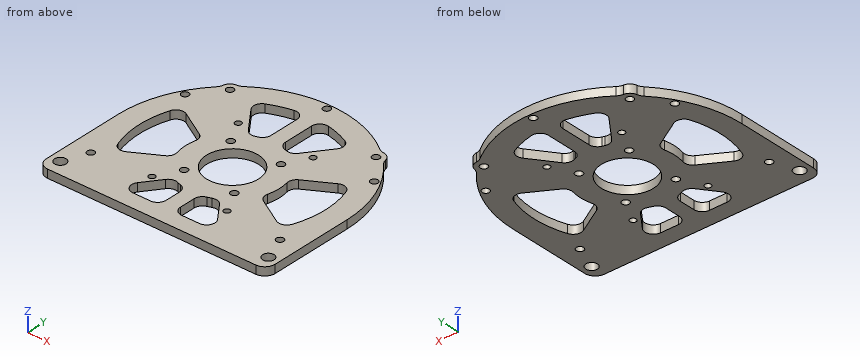
```python
from build123d import *

# Parameters (mm, degrees)
SKETCH_2_R          = 1.25
SKETCH_2_R_2        = 1.75
SKETCH_2_R_3        = 12.5
SKETCH_2_R_4        = 2.55
SKETCH_2_R_5        = 1.5
SKETCH_2_R_6        = 1.55
EXTRUDE_1_DEPTH     = 4
CUT_EXTRUDE_1_DEPTH = 4
FILLET_2_R          = 4
FILLET_3_R          = 4
FILLET_4_R          = 5
SKETCH_4_R          = 1.75
SKETCH_4_R_2        = 1.5
SKETCH_4_R_3        = 2.75
CUT_EXTRUDE_2_DEPTH = 10


with BuildPart() as part:
    # 草图2 → 凸台-拉伸1 (new body)
    with BuildSketch(Plane.XY):
        with BuildLine():
            Line((55, 3), (55, 47.999999928))
            ThreePointArc((55, 47.999999928), (50.85407892, 68.949049075), (39.041357871, 86.739803505))
            ThreePointArc((39.041357871, 86.739803505), (37.739334229, 90.232640986), (34.122629592, 91.135207774))
            ThreePointArc((34.122629592, 91.135207774), (0, 103), (-34.122629592, 91.135207774))
            ThreePointArc((-34.122629592, 91.135207774), (-37.739334229, 90.232640986), (-39.041357871, 86.739803505))
            ThreePointArc((-39.041357871, 86.739803505), (-50.854078907, 68.949049108), (-55, 48))
            Line((-55, 48), (-55, 3))
            Line((-55, 3), (55, 3))
        make_face()
        with Locations((-18, 24)):
            Circle(SKETCH_2_R, mode=Mode.SUBTRACT)
        with Locations((-12.07, 35)):
            Circle(SKETCH_2_R_2, mode=Mode.SUBTRACT)
        with Locations((18, 24)):
            Circle(SKETCH_2_R, mode=Mode.SUBTRACT)
        with Locations((12.07, 35)):
            Circle(SKETCH_2_R_2, mode=Mode.SUBTRACT)
        with Locations((0, 48)):
            Circle(SKETCH_2_R_3, mode=Mode.SUBTRACT)
        with Locations((-12.07, 61)):
            Circle(SKETCH_2_R_2, mode=Mode.SUBTRACT)
        with Locations((-18, 72)):
            Circle(SKETCH_2_R, mode=Mode.SUBTRACT)
        with Locations((12.07, 61)):
            Circle(SKETCH_2_R_2, mode=Mode.SUBTRACT)
        with Locations((18, 72)):
            Circle(SKETCH_2_R, mode=Mode.SUBTRACT)
        with Locations((50, 10)):
            Circle(SKETCH_2_R_4, mode=Mode.SUBTRACT)
        with Locations((45.466333699, 21.75)):
            Circle(SKETCH_2_R_5, mode=Mode.SUBTRACT)
        with Locations((45.466333699, 74.25)):
            Circle(SKETCH_2_R_5, mode=Mode.SUBTRACT)
        with Locations((35.074028853, 87.25)):
            Circle(SKETCH_2_R_6, mode=Mode.SUBTRACT)
        with Locations((-50, 10)):
            Circle(SKETCH_2_R_4, mode=Mode.SUBTRACT)
        with Locations((0, 100.5)):
            Circle(SKETCH_2_R_5, mode=Mode.SUBTRACT)
        with Locations((-45.466333699, 21.75)):
            Circle(SKETCH_2_R_5, mode=Mode.SUBTRACT)
        with Locations((-45.466333699, 74.25)):
            Circle(SKETCH_2_R_5, mode=Mode.SUBTRACT)
        with Locations((-35.074028853, 87.25)):
            Circle(SKETCH_2_R_6, mode=Mode.SUBTRACT)
    extrude(amount=EXTRUDE_1_DEPTH)

    # 草图3 → 切除-拉伸1 (cut)
    with BuildSketch(Plane.XY.offset(4)):
        with BuildLine():
            ThreePointArc((-3.5, 25.773889229), (-7.354360894, 26.735866445), (-10.979461873, 28.360717503))
            Line((-10.979461873, 28.360717503), (-24, 11))
            Line((-24, 11), (-3.5, 11))
            Line((-3.5, 11), (-3.5, 25.773889229))
        make_face()
        with BuildLine():
            Line((-21.175179269, 55.606693298), (-40.502045801, 66.765064893))
            ThreePointArc((-40.502045801, 66.765064893), (-44.635096369, 47.4984557), (-40.070163739, 28.329581794))
            Line((-40.070163739, 28.329581794), (-20.811589784, 39.448524651))
            ThreePointArc((-20.811589784, 39.448524651), (-22.494305888, 47.493835393), (-21.175179269, 55.606693298))
        make_face()
        with BuildLine():
            ThreePointArc((-3.5, 92.500487352), (-13.877512662, 90.425912092), (-23.474999809, 85.966666412))
            Line((-23.474999809, 85.966666412), (-10.084953895, 68.11327186))
            ThreePointArc((-10.084953895, 68.11327186), (-6.874137411, 69.424197414), (-3.5, 70.226110771))
            Line((-3.5, 70.226110771), (-3.5, 92.500487352))
        make_face()
    cut_extrude_1 = extrude(amount=-CUT_EXTRUDE_1_DEPTH, mode=Mode.SUBTRACT)

    # 镜向1: 切除-拉伸1 across plane
    add(cut_extrude_1.mirror(Plane(origin=(0, 0, 0), x_dir=(0, 0, 1), z_dir=(1, 0, 0))), mode=Mode.SUBTRACT)

    # 圆角2
    fillet_2_edges = [part.edges().sort_by_distance(p)[0] for p in [
        (-40.502045801, 66.765064893, 2),
        (-21.175179269, 55.606693298, 2),
        (-20.811589784, 39.448524651, 2),
        (-40.070163739, 28.329581794, 2),
    ]]
    fillet(fillet_2_edges, radius=FILLET_2_R)

    # 圆角3
    fillet_3_edges = [part.edges().sort_by_distance(p)[0] for p in [
        (-3.5, 92.500487352, 2),
        (-3.5, 70.226110771, 2),
        (-10.084953895, 68.11327186, 2),
        (-23.474999809, 85.966666412, 2),
        (-10.979461873, 28.360717503, 2),
        (-3.5, 25.773889229, 2),
        (-3.5, 11, 2),
        (-24, 11, 2),
        (3.5, 70.226110771, 2),
        (3.5, 92.500487352, 2),
        (23.474999809, 85.966666412, 2),
        (10.084953895, 68.11327186, 2),
        (21.175179269, 55.606693298, 2),
        (40.502045801, 66.765064893, 2),
        (40.070163739, 28.329581794, 2),
        (20.811589784, 39.448524651, 2),
        (3.5, 25.773889229, 2),
        (10.979461873, 28.360717503, 2),
        (24, 11, 2),
        (3.5, 11, 2),
    ]]
    fillet(fillet_3_edges, radius=FILLET_3_R)

    # 圆角4
    fillet_4_edges = [part.edges().sort_by_distance(p)[0] for p in [
        (39.041357871, 86.739803505, 2),
        (55, 3, 2),
        (-55, 3, 2),
        (-39.041357871, 86.739803505, 2),
        (-34.122629592, 91.135207774, 2),
        (34.122629592, 91.135207774, 2),
    ]]
    fillet(fillet_4_edges, radius=FILLET_4_R)

    # 草图4 → 切除-拉伸2 (cut)
    with BuildSketch(Plane.XY.offset(4)):
        with Locations((-45.466333699, 74.25)):
            Circle(SKETCH_4_R)
        with Locations((-35.074028853, 87.25)):
            Circle(SKETCH_4_R)
        with Locations((0, 100.5)):
            Circle(SKETCH_4_R)
        with Locations((35.074028853, 87.25)):
            Circle(SKETCH_4_R)
        with Locations((45.466333699, 74.25)):
            Circle(SKETCH_4_R)
        with Locations((18, 72)):
            Circle(SKETCH_4_R_2)
        with Locations((-18, 72)):
            Circle(SKETCH_4_R_2)
        with Locations((-18, 24)):
            Circle(SKETCH_4_R_2)
        with Locations((18, 24)):
            Circle(SKETCH_4_R_2)
        with Locations((50, 10)):
            Circle(SKETCH_4_R_3)
        with Locations((-50, 10)):
            Circle(SKETCH_4_R_3)
        with Locations((45.466333699, 21.75)):
            Circle(SKETCH_4_R)
        with Locations((-45.466333699, 21.75)):
            Circle(SKETCH_4_R)
    extrude(amount=-CUT_EXTRUDE_2_DEPTH, mode=Mode.SUBTRACT)


solid = part.part
```
Source: CAD feature listing. Evaluate the final solid. Frame: model axes, mm. Round coordinates to 2 decimals unless told otherwise and drop trailing zeros. Write each loop counter-clockwise with the first axis right and the second up, starting at its lowest first coordinate (ties: lowest second). Pieces come first, ordered by that corner, then holes. Notation, with made-up numbers: M 85.5,71 L 138.5,71 A23 ccw 138.5,102 Z; hole C -16.75,89 d4. An arc over 180 degrees is marked long. Use CSV: the item, a comma, the result in double quotes. Start each with the question number.
Q1. Cut plane A-A on x = 0. Output: boundary loops of the cut face in (y, z).
Q2. Cut plane B-B on x = -18. Output: boundary loops of the cut face in (y, z).
Q3. First-contact query: P1, Ø6, axis at x = -24.5, y = 57.5, coming from the +Z side; P2, Ø2, axis at x = 45.47, y = 21.75, coming from the +Z side; P3, Ø1.2, axis at y = 77.5, z = 1, coming from the +X side; P4, Ø1, axis at y = 87, z = 2, coming from the -X side. Flat tips, straight axial feed; report the tip coordinate or a pass-through.
Q4. Cut plane D-D on y = 94.5. Output: boundary loops of the cut face in (x, z), plus the area to 3 significant figures.
Q5. Line query: line 1 (X direction, y = 8, z = 2.7); line 2 (Y direction, x = 18, z = 2.25); line 3 (X direction, y = 64.5, z = 1.65). Output: solid intervals per line, ascending. Write a range as from..to.
Q6. Cut plane C-C on z = 2.65. Count the separate pieces of the cut face and the enclosed holes in it, plus the area to 3 significant figures.
Results found:
1,outline,"M 3,0 L 35.5,0 L 35.5,4 L 3,4 Z; M 60.5,0 L 98.75,0 L 98.75,4 L 60.5,4 Z; M 102.25,0 L 103,0 L 103,4 L 102.25,4 Z"
2,outline,"M 3,0 L 11.54,0 L 11.54,4 L 3,4 Z; M 19,0 L 22.5,0 L 22.5,4 L 19,4 Z; M 25.5,0 L 70.5,0 L 70.5,4 L 25.5,4 Z; M 73.5,0 L 78.67,0 L 78.67,4 L 73.5,4 Z; M 88.85,0 L 99.97,0 L 99.97,4 L 88.85,4 Z"
3,P1,"z = 4"
3,P2,"through"
3,P3,"x = 46.8"
3,P4,"x = -39.52"
4,outline,"M -29.37,0 L 29.37,0 L 29.37,4 L -29.37,4 Z"
4,area,"235 mm^2"
5,line 1,"-55..-51.89, -48.11..48.11, 51.89..55"
5,line 2,"3..11.54, 19..22.5, 25.5..70.5, 73.5..78.67, 88.85..99.97"
5,line 3,"-52.47..-40.43, -36.58..36.58, 40.43..52.47"
6,separate pieces,"1"
6,enclosed holes,"24"
6,area,"6,800 mm^2"
